```python
from build123d import *

# Parameters (mm, degrees)
SKETCH1_R                = 97
SKETCH1_R_2              = 59.5
BASE_DEPTH               = 5
TANG_START               = -5
TANG_DEPTH               = 5
FILLET1_R                = 8
CIRPATTERN1_COUNT        = 3
FILLET1_OF_CIRPATTERN1_R = 8


with BuildPart() as part:
    # Sketch1 → Base (new body)
    with BuildSketch(Plane.XY):
        Circle(SKETCH1_R)
        Circle(SKETCH1_R_2, mode=Mode.SUBTRACT)
    extrude(amount=BASE_DEPTH)

    # Sketch2 → Tang (add)
    with BuildSketch(Plane.XY.offset(5).offset(TANG_START)):
        with BuildLine():
            Line((-95.802126652, 50.60091431), (-86.427728757, 44.036890238))
            ThreePointArc((-86.427728757, 44.036890238), (-79.457748296, 55.636914326), (-70.941164976, 66.153995434))
            Line((-70.941164976, 66.153995434), (-80.31556287, 72.718019506))
            ThreePointArc((-80.31556287, 72.718019506), (-99.117397359, 69.402748798), (-95.802126652, 50.60091431))
        make_face()
    tang = extrude(amount=TANG_DEPTH)

    # Fillet1
    fillet1_edges = [part.edges().sort_by_distance(p)[0] for p in [
        (-70.941164976, 66.153995434, 2.5),
        (-86.427728757, 44.036890238, 2.5),
    ]]
    fillet(fillet1_edges, radius=FILLET1_R)

    # Sketch3 → M5x0.8 Tapped Hole1 (revolve, cut)
    with BuildSketch(Plane(origin=(-88.058844761, 61.659466908, 5), x_dir=(0, -1, 0), z_dir=(1, 0, 0))):
        Polygon((0, 0), (0, 5), (3, 5), (2.1, 4.1), (2.1, 0.9), (3, 0), align=None)
    m5x0_8_tapped_hole1 = revolve(axis=Axis((-88.058844761, 61.659466908, 11.35), (0, 0, -1)), mode=Mode.SUBTRACT)

    # CirPattern1: Tang, M5x0.8 Tapped Hole1 ×3 about axis
    cirpattern1_axis = Axis((0, 0, 0), (0, 0, 1))
    add([tang.rotate(cirpattern1_axis, i * 360 / CIRPATTERN1_COUNT) for i in range(1, CIRPATTERN1_COUNT)])
    add([m5x0_8_tapped_hole1.rotate(cirpattern1_axis, i * 360 / CIRPATTERN1_COUNT) for i in range(1, CIRPATTERN1_COUNT)], mode=Mode.SUBTRACT)

    # Fillet1 of CirPattern1
    fillet1_of_cirpattern1_edges = [part.edges().sort_by_distance(p)[0] for p in [
        (-21.82045812, -94.51384876, 2.5),
        (5.076798729, -96.867053814, 2.5),
        (92.761623095, 28.359853326, 2.5),
        (81.350930028, 52.830163576, 2.5),
    ]]
    fillet(fillet1_of_cirpattern1_edges, radius=FILLET1_OF_CIRPATTERN1_R)


solid = part.part
```
Source: CAD feature listing. Evaluate the final solid. Frame: model axes, mm. A direction names the side the tool comes from. Coordinates: 2 decimals unless noted, no trailing zeros. Loops run counter-clockwise (first coordinate to the right, second up) from the corner with the lowest first, then second, coordinate; pieces in that order, holes last. Notation, with made-up numbers: (-38.75, -0.75) - (2.25, -0.75) arc R9 cw to (2.25, 15.25) - close; hole circle Ø5 at (-22, 27). An arc over 180 degrees is marked (long way). Answer as CSV lines item,"result".
1. Section C-C (z = 2.7). Return loops of the section in (x, y).
Established:
outline,"(-95.8, 50.6) - (-91.93, 47.89) arc R8 cw to (-89.17, 38.19) arc R97 ccw to (-28.06, -92.85) arc R8 cw to (-22.41, -101.21) - (-22.82, -105.91) arc R13.5 ccw to (4.08, -108.27) - (4.49, -103.56) arc R8 cw to (11.51, -96.31) arc R97 ccw to (94.44, 22.12) arc R8 cw to (98.85, 31.2) - (103.13, 33.2) arc R13.5 ccw to (91.72, 57.67) - (87.44, 55.67) arc R8 cw to (77.66, 58.13) arc R97 ccw to (-66.38, 70.73) arc R8 cw to (-76.45, 70.01) - (-80.32, 72.72) arc R13.5 ccw to start; hole circle Ø4.2 at (-88.06, 61.66); hole circle Ø119 at (0, 0); hole circle Ø4.2 at (-9.37, -107.09); hole circle Ø4.2 at (97.43, 45.43)"
2. Section A-A (y = 0). Return loops of the section in (x, z).
Established:
outline,"(-97, 0) - (-59.5, 0) - (-59.5, 5) - (-97, 5) - close; (59.5, 0) - (97, 0) - (97, 5) - (59.5, 5) - close"
3. Ray query, line 1 (Y direction, x = 0, z = 2.2); line 2 (Y direction, x = 15.5, z = 1.8); line 3 (X direction, y = -44, z = 0.5). Return the intervals inside material, ascending.
Established:
line 1,"y = -116.81 to -59.5, 59.5 to 97"
line 2,"y = -95.75 to -57.45, 57.45 to 95.75"
line 3,"x = -86.45 to -40.05, 40.05 to 86.45"
4. Reachability of faces 1 (the cylindrical face through (-71.21, 68.587, 2.535)), 2 (the flat face through (-22.61, -103.53, 2.46)) from +Z, -Z, +X, -X, +Y, -Y: full face, straight path, thin tool, end or side. Return the list, or none.
Established:
face 1,"+Z, -Z, +Y"
face 2,"+Z, -Z, -X"
5. Section D-D (y = -69). Return loops of the section in (x, z).
Established:
outline,"(-68.18, 0) - (68.18, 0) - (68.18, 5) - (-68.18, 5) - close"
6. Mould query, pull axis Y, two halves, no side actions, for faces 3 (the cylindrical face through (82.04, 55.18, 2.54)), 4 (the cylindrical face through (6.768, -98.637, 2.535)), 5 (the cylindrical face through (-23.794, -95.963, 2.535)). Classes: released by +Y, released by -Y, zero draft, split by the parting line, or undercut.
Established:
face 3,"released by +Y"
face 4,"released by -Y"
face 5,"undercut"
7. Contact query for flat-ended pins moving along their axis: pin 1 (3 mm diameter, centred on x = -39.5, z = 3, fed in from -Y); pin 2 (1 mm diameter, centred on y = -14, z = 2, fed in from -X); pin 3 (6.5 mm diameter, centred on x = -88.06, y = 61.66, fed in from +Z); pin 4 (4 mm diameter, centred on x = -9.37, y = -107.09, fed in from +Z). Output: stop coordinate, or through.
Established:
pin 1,"stops at y = -89.25"
pin 2,"stops at x = -96.06"
pin 3,"stops at z = 5"
pin 4,"passes through"
8. Section B-B (x = 0). Return loops of the section in (y, z), then the cut area to 3 significant figures.
Established:
outline,"(-116.81, 0) - (-59.5, 0) - (-59.5, 5) - (-116.81, 5) - close; (59.5, 0) - (97, 0) - (97, 5) - (59.5, 5) - close"
area,"474 mm2"
